Read the model definition and answer for the solid it produces. Units are mm, in the model's axes. Give positions to 0.01 mm unless a question says otherwise; leave off trailing zeros. Write each loop counter-clockwise with the first axis right and the second up, starting at its lowest first coordinate (ties: lowest second). Pieces come first, ordered by that corner, then holes. Notation, with made-up numbers: (-26.5, 11) -> (8.5, 11) arc R13 ccw to (8.5, 29) -> close; hole circle Ø9 at (74, -21.75). An arc over 180 degrees is marked (long way). Answer as CSV lines item,"result". Start each with the question number.
1. Find the intervals of material crossed by line 1 (Z direction, x = 264, y = -53.5); line 2 (Y direction, x = 1067.5, z = -75.5); line 3 (X direction, y = -57.5, z = -16), in increasing order.
2. The part is cut by section B-B, the plane y = -36. Determine the outline of the cut face in (x, z), and give its area (3 significant figures).
3. The part is cut by section A-A, the plane x = 827. Determine the outline of the cut face in (y, z), and give its area (3 significant figures).
4. Given pin 1 (14 mm diameter, centred on x = 914, z = -66, fed in from -Y); pin 2 (4 mm diameter, centred on x = 1196.5, y = -23, fed in from +Z); pin 3 (10 mm diameter, centred on x = 865.5, y = -24.5, fed in from -Z); pin 4 (7 mm diameter, centred on x = 424, z = -66, fed in from -Y), each flat-ended and moving along its own axis, determine where each tip first touches the part or whether it passes through.
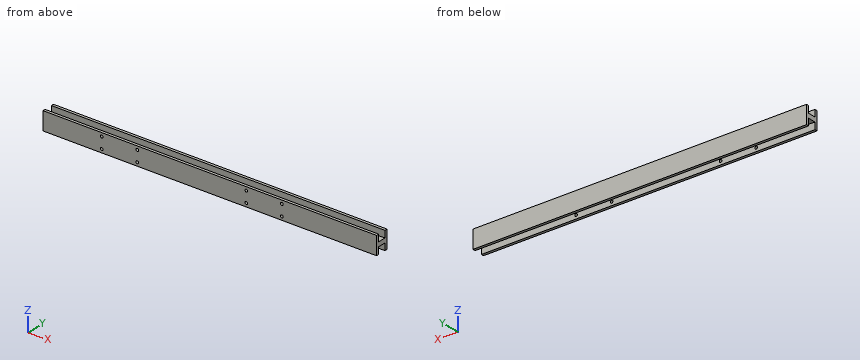
from build123d import *

# Parameters (mm, degrees)
BOSS_EXTRUDE1_DEPTH            = 1500
CUT_EXTRUDE1_REACH             = 1505.437
SKETCH4_R                      = 6
CUT_EXTRUDE1_DIRECTION_2_DEPTH = 1504.437394772


with BuildPart() as part:
    # Sketch1 → Boss-Extrude1 (new body)
    with BuildSketch(Plane(origin=(0, 0, 0), x_dir=(0, 0, -1), z_dir=(1, 0, 0))):
        Polygon((51, -12), (82, -12), (82, 0), (0, 0), (0, -12), (31, -12), (31, -48), (0, -48), (0, -60), (82, -60), (82, -48), (51, -48), align=None)
    extrude(amount=BOSS_EXTRUDE1_DEPTH)

    # Sketch4 → Cut-Extrude1 (cut, up to next)
    with BuildSketch(Plane(origin=(0, -60, 0), x_dir=(-1, 0, 0), z_dir=(0, -1, 0)), mode=Mode.PRIVATE) as cut_extrude1_sk1:
        with Locations(Location((-424, 16, 0), (0, 0, 270))):
            Circle(SKETCH4_R)
    cut_extrude1_tool1 = extrude(cut_extrude1_sk1.sketch, amount=-CUT_EXTRUDE1_REACH, mode=Mode.PRIVATE) & part.part
    # Sketch4 → Cut-Extrude1 (cut, up to next)
    with BuildSketch(Plane(origin=(0, -60, 0), x_dir=(-1, 0, 0), z_dir=(0, -1, 0)), mode=Mode.PRIVATE) as cut_extrude1_sk2:
        with Locations(Location((-424, 66, 0), (0, 0, 270))):
            Circle(SKETCH4_R)
    cut_extrude1_tool2 = extrude(cut_extrude1_sk2.sketch, amount=-CUT_EXTRUDE1_REACH, mode=Mode.PRIVATE) & part.part
    # Sketch4 → Cut-Extrude1 (cut, up to next)
    with BuildSketch(Plane(origin=(0, -60, 0), x_dir=(-1, 0, 0), z_dir=(0, -1, 0)), mode=Mode.PRIVATE) as cut_extrude1_sk3:
        with Locations(Location((-264, 66, 0), (0, 0, 270))):
            Circle(SKETCH4_R)
    cut_extrude1_tool3 = extrude(cut_extrude1_sk3.sketch, amount=-CUT_EXTRUDE1_REACH, mode=Mode.PRIVATE) & part.part
    # Sketch4 → Cut-Extrude1 (cut, up to next)
    with BuildSketch(Plane(origin=(0, -60, 0), x_dir=(-1, 0, 0), z_dir=(0, -1, 0)), mode=Mode.PRIVATE) as cut_extrude1_sk4:
        with Locations(Location((-264, 16, 0), (0, 0, 270))):
            Circle(SKETCH4_R)
    cut_extrude1_tool4 = extrude(cut_extrude1_sk4.sketch, amount=-CUT_EXTRUDE1_REACH, mode=Mode.PRIVATE) & part.part
    # Sketch4 → Cut-Extrude1 (cut, up to next)
    with BuildSketch(Plane(origin=(0, -60, 0), x_dir=(-1, 0, 0), z_dir=(0, -1, 0)), mode=Mode.PRIVATE) as cut_extrude1_sk5:
        with Locations(Location((-1074, 66, 0), (0, 0, 270))):
            Circle(SKETCH4_R)
    cut_extrude1_tool5 = extrude(cut_extrude1_sk5.sketch, amount=-CUT_EXTRUDE1_REACH, mode=Mode.PRIVATE) & part.part
    # Sketch4 → Cut-Extrude1 (cut, up to next)
    with BuildSketch(Plane(origin=(0, -60, 0), x_dir=(-1, 0, 0), z_dir=(0, -1, 0)), mode=Mode.PRIVATE) as cut_extrude1_sk6:
        with Locations(Location((-914, 66, 0), (0, 0, 270))):
            Circle(SKETCH4_R)
    cut_extrude1_tool6 = extrude(cut_extrude1_sk6.sketch, amount=-CUT_EXTRUDE1_REACH, mode=Mode.PRIVATE) & part.part
    # Sketch4 → Cut-Extrude1 (cut, up to next)
    with BuildSketch(Plane(origin=(0, -60, 0), x_dir=(-1, 0, 0), z_dir=(0, -1, 0)), mode=Mode.PRIVATE) as cut_extrude1_sk7:
        with Locations(Location((-1074, 16, 0), (0, 0, 270))):
            Circle(SKETCH4_R)
    cut_extrude1_tool7 = extrude(cut_extrude1_sk7.sketch, amount=-CUT_EXTRUDE1_REACH, mode=Mode.PRIVATE) & part.part
    # Sketch4 → Cut-Extrude1 (cut, up to next)
    with BuildSketch(Plane(origin=(0, -60, 0), x_dir=(-1, 0, 0), z_dir=(0, -1, 0)), mode=Mode.PRIVATE) as cut_extrude1_sk8:
        with Locations(Location((-914, 16, 0), (0, 0, 270))):
            Circle(SKETCH4_R)
    cut_extrude1_tool8 = extrude(cut_extrude1_sk8.sketch, amount=-CUT_EXTRUDE1_REACH, mode=Mode.PRIVATE) & part.part
    add(cut_extrude1_tool1.solids().sort_by_distance((424, -60, -16))[0], mode=Mode.SUBTRACT)
    add(cut_extrude1_tool2.solids().sort_by_distance((424, -60, -66))[0], mode=Mode.SUBTRACT)
    add(cut_extrude1_tool3.solids().sort_by_distance((264, -60, -66))[0], mode=Mode.SUBTRACT)
    add(cut_extrude1_tool4.solids().sort_by_distance((264, -60, -16))[0], mode=Mode.SUBTRACT)
    add(cut_extrude1_tool5.solids().sort_by_distance((1074, -60, -66))[0], mode=Mode.SUBTRACT)
    add(cut_extrude1_tool6.solids().sort_by_distance((914, -60, -66))[0], mode=Mode.SUBTRACT)
    add(cut_extrude1_tool7.solids().sort_by_distance((1074, -60, -16))[0], mode=Mode.SUBTRACT)
    add(cut_extrude1_tool8.solids().sort_by_distance((914, -60, -16))[0], mode=Mode.SUBTRACT)

    # Sketch4 → Cut-Extrude1 direction 2 (cut)
    with BuildSketch(Plane(origin=(0, -60, 0), x_dir=(-1, 0, 0), z_dir=(0, -1, 0))):
        with Locations(Location((-424, 16, 0), (0, 0, 270))):
            Circle(SKETCH4_R)
        with Locations(Location((-424, 66, 0), (0, 0, 270))):
            Circle(SKETCH4_R)
        with Locations(Location((-264, 66, 0), (0, 0, 270))):
            Circle(SKETCH4_R)
        with Locations(Location((-264, 16, 0), (0, 0, 270))):
            Circle(SKETCH4_R)
        with Locations(Location((-1074, 66, 0), (0, 0, 270))):
            Circle(SKETCH4_R)
        with Locations(Location((-914, 66, 0), (0, 0, 270))):
            Circle(SKETCH4_R)
        with Locations(Location((-1074, 16, 0), (0, 0, 270))):
            Circle(SKETCH4_R)
        with Locations(Location((-914, 16, 0), (0, 0, 270))):
            Circle(SKETCH4_R)
    extrude(amount=CUT_EXTRUDE1_DIRECTION_2_DEPTH, mode=Mode.SUBTRACT)


solid = part.part
Results found:
1,line 1,"z = -82 to -72, -60 to -22, -10 to 0"
1,line 2,"y = -60 to -48, -12 to 0"
1,line 3,"x = 0 to 258, 270 to 418, 430 to 908, 920 to 1068, 1080 to 1500"
2,outline,"(0, -51) -> (1500, -51) -> (1500, -31) -> (0, -31) -> close"
2,area,"30,000 mm²"
3,outline,"(-60, -82) -> (-48, -82) -> (-48, -51) -> (-12, -51) -> (-12, -82) -> (0, -82) -> (0, 0) -> (-12, 0) -> (-12, -31) -> (-48, -31) -> (-48, 0) -> (-60, 0) -> close"
3,area,"2,690 mm²"
4,pin 1,"stops at y = -60"
4,pin 2,"stops at z = -31"
4,pin 3,"stops at z = -51"
4,pin 4,"stops at y = -12"
